Read the model definition and answer for the solid it produces. Units are mm, in the model's axes. Coordinates: 2 decimals unless noted, no trailing zeros. Write each loop counter-clockwise with the first axis right and the second up, starting at its lowest first coordinate (ties: lowest second). Pieces come first, ordered by that corner, then holes. Notation, with made-up numbers: (20.25, 23) -> (40.25, 23) arc R9 cw to (40.25, 27) -> close; hole circle Ø8 at (75, 15). An arc over 180 degrees is marked (long way). One line per item, written item: value. Start each with the question number.
Autodesk Inventor part; units mm, degrees
ref_plane "YZ Plane" through (0, 0, 0) normal (1, 0, 0) x (0, 1, 0)
ref_plane "XZ Plane" through (0, 0, 0) normal (0, 1, 0) x (-1, 0, 0)
ref_plane "XY Plane" through (0, 0, 0) normal (0, 0, 1) x (1, 0, 0)
sketch "Esboço1" plane through (0, 0, 0) normal (0, 0, 1) x (1, 0, 0)
  arc A0 (4, 2.4377) -> (-4, 2.4377) centre (0, 9.3659) ccw
  line L0 (9.25, -3.9341) -> (9.25, -10.6341)
  line L1 (-9.25, -10.6341) -> (-9.25, -3.9341)
  line L2 (4, -15.6341) -> (-4, -15.6341)
  line L3 (20, -15.6341) -> (-20, -15.6341)
  line L4 (-20, -15.6341) -> (-20, -10.6341)
  line L5 (20, -10.6341) -> (20, -15.6341)
  line L6 (7.6788, -3.9341) -> (9.25, -3.9341)
  line L7 (-9.25, -3.9341) -> (-7.6788, -3.9341)
  line L8 (9.25, -10.6341) -> (20, -10.6341)
  line L9 (-20, -10.6341) -> (-9.25, -10.6341)
  line L10 (-4, 2.4377) -> (-7.6788, -3.9341)
  line L11 (-17.4151, -20.798) -> (-22.4188, -29.4646)
  line L12 (17.4151, -20.798) -> (23.6527, -31.6017)
  line L13 (9.25, -15.6341) -> (4, -15.6341)
  line L14 (0, -15.6341) -> (-9.25, -15.6341)
  line L15 (4, 2.4377) -> (7.6788, -3.9341)
  dimension "d6" = 16
  dimension "d7" = 25
  dimension "d8" = 18.5
  dimension "d9" = 11.7
  dimension "d10" = 8
  dimension "d13" = 5
  dimension "d14" = 40
extrude "Extrusão1" add sketch "Esboço1" along normal blind 1054
sketch "Esboço3" plane through (-20, -15.6341, 0) normal (0, -1, 0) x (1, 0, 0)
  line L0 (0, 1054) -> (40, 1054) construction
  line L1 (20, 1054) -> (20, 0) construction
  line L2 (20, 1029) -> (5, 1029) construction
  line L3 (5, 1029) -> (20, 1029) construction
  line L4 (20, 1029) -> (35, 1029) construction
  circle A0 centre (5, 1029) radius 2.75
  circle A1 centre (35, 1029) radius 2.75
  line L5 (40, 0) -> (0, 0) construction
  line L6 (35, 1054) -> (35, 0) construction
  line L7 (5, 1054) -> (5, 0) construction
  point P0 (5, 879)
  point P1 (35, 879)
  point P2 (5, 729)
  point P3 (35, 729)
  point P4 (5, 579)
  point P5 (35, 579)
  point P6 (5, 429)
  point P7 (35, 429)
  point P8 (5, 279)
  point P9 (35, 279)
  point P10 (5, 129)
  point P11 (35, 129)
  dimension "d18" = 15
  dimension "d19" = 15
  dimension "d20" = 5.5
  dimension "d21" = 5.5
  dimension "d22" = 25
  dimension "d39" = 150
hole "Furo2" at (-15, -15.6341, 279) at (15, -15.6341, 279) at (15, -15.6341, 129) at (-15, -15.6341, 129) at (15, -15.6341, 429) at (-15, -15.6341, 429) at (15, -15.6341, 579) at (-15, -15.6341, 579) at (15, -15.6341, 729) at (-15, -15.6341, 729) at (-15, -15.6341, 879) at (15, -15.6341, 879) at (15, -15.6341, 1029) at (-15, -15.6341, 1029) direction (0, 1, 0) diameter 5.5 end through all
properties part number "SBR16_EIXO_Y_1"
1. A cutting plane is placed at B-B on y = 11.5. Give the vertices of the cut face in (x, z).
2. A cutting plane is placed at A-A on z = 324. Give the vertices of the cut face in (x, y), then the cut area to 3 significant figures.
3. Find the intervals of material crossed by probe 1 along X at (y, z) = (-13, 579); probe 2 along X at (y, z) = (10.5, 942); probe 3 along X at (y, z) = (11.5, 97), in increasing order. Write a range as from..to.
4. Given pin 1 (6.5 mm diameter, centred on x = 15, z = 879, fed in from -Y); pin 2 (1 mm diameter, centred on y = 9.5, z = 871.5, fed in from +X); pin 3 (7 mm diameter, centred on x = -15, z = 729, fed in from +Y); pin 4 (1.5 mm diameter, centred on y = 1, z = 840, fed in from +X), each flat-ended and moving along its own axis, determine where each tip first touches the part or whether it passes through.
Derived:
1. outline: (-7.71, 0) -> (7.71, 0) -> (7.71, 1054) -> (-7.71, 1054) -> close
2. outline: (-20, -15.63) -> (20, -15.63) -> (20, -10.63) -> (9.25, -10.63) -> (9.25, -3.93) -> (7.68, -3.93) -> (4, 2.44) arc R8 ccw (long way) to (-4, 2.44) -> (-7.68, -3.93) -> (-9.25, -3.93) -> (-9.25, -10.63) -> (-20, -10.63) -> close
2. area: 594 mm2
3. probe 1: x = -20..-17.75, -12.25..12.25, 17.75..20
3. probe 2: x = -7.92..7.92
3. probe 3: x = -7.71..7.71
4. pin 1: stops at y = -15.63
4. pin 2: stops at x = 8
4. pin 3: stops at y = -10.63
4. pin 4: stops at x = 5.26
